Design review of the part shown in the three views and the two pictorial views. Dimensions are in mm from the part's minimum x, y and z. Coordinates: 2 decimals unless noted, no trailing zeros. Loops run counter-clockwise (first coordinate to the right, second up) from the corner with the lowest first, then second, coordinate; pieces in that order, holes last. Notation, with made-up numbers: M -21.5,36.25 L -6.5,36.25 A23 cw -6.5,61.25 Z; hole C 36,35 d1. An arc over 180 degrees is marked long. Put each result on its own line as item: value. Start each with the question number.
(1) Take a section at C-C, the plane y = 74.5. Give the boundary of the cut face in (x, z), then the cut area to 3 significant figures.
(2) Take a section at A-A, the plane x = 10.75. Give the boundary of the cut face in (y, z).
(3) Take a section at B-B, the plane y = 40. Give the boundary of the cut face in (x, z), then the cut area to 3 significant figures.
(4) Take a section at D-D, the plane z = 221. Give the boundary of the cut face in (x, y).
(5) For probe 1 along Y at (x, z) = (15.75, 58.5); probe 2 along Y at (x, z) = (14.5, 210); probe 3 along Y at (x, z) = (4.25, 26.5), list the stretches that pass through material, from the lowest coordinate up. Write a range as [from, to].
(6) Clearance check with flat-ended pins moving along their axes: pin 1 (11 mm diameter, centred on y = 40, z = 210, fed in from +X); pin 2 (16 mm diameter, centred on x = 17, y = 41, fed in from +Z); pin 3 (2 mm diameter, centred on x = 18.5, y = 37, fed in from +Z); pin 4 (5 mm diameter, centred on x = 12, y = 29.5, fed in from -Z). State where each tip first meets the part, or that it passes through.
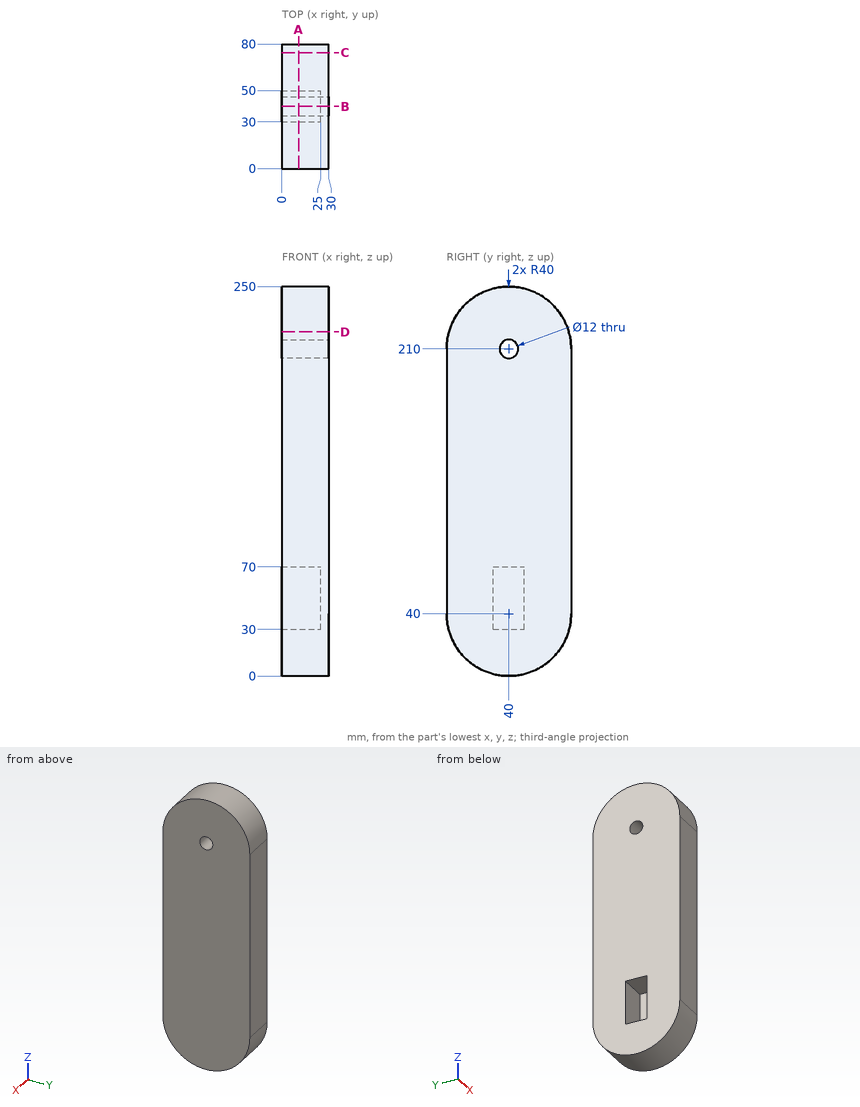
Computed values:
1. outline: M 0,19.76 L 30,19.76 L 30,230.24 L 0,230.24 Z
1. area: 6,310 mm^2
2. outline: M 0,40 A40 ccw 80,40 L 80,210 A40 ccw 0,210 Z; hole M 30,30 L 50,30 L 50,70 L 30,70 Z; hole C 40,210 d12
3. outline: M 0,0 L 30,0 L 30,204 L 0,204 L 0,70 L 25,70 L 25,30 L 0,30 Z; M 0,216 L 30,216 L 30,250 L 0,250 Z
3. area: 6,140 mm^2
4. outline: M 0,1.54 L 30,1.54 L 30,78.46 L 0,78.46 Z
5. probe 1: y = [0, 30], [50, 80]
5. probe 2: y = [0, 34], [46, 80]
5. probe 3: y = [2.35, 77.65]
6. pin 1: passes through
6. pin 2: stops at z = 250
6. pin 3: stops at z = 249.95
6. pin 4: stops at z = 0.81
